Autodesk Fusion 360 part; units mm, degrees
sketch "Sketch1" plane through (0, 0, 0) normal (0, 1, 0) x (1, 0, 0)
  line L0 (17.145, 0) -> (68.58, 0)
  line L1 (91.44, 22.86) -> (91.44, 109.855)
  line L2 (74.295, 127) -> (22.86, 127)
  line L3 (0, 104.14) -> (0, 17.145)
  circle A0 centre (12.7, 31.75) radius 1.905
  circle A1 centre (78.74, 95.25) radius 1.905
  circle A2 centre (78.74, 31.75) radius 1.905
  circle A3 centre (12.7, 95.25) radius 1.905
  circle A4 centre (28.525, 20.96) radius 1.375
  circle A5 centre (62.915, 20.96) radius 1.375
  circle A6 centre (62.915, 106.04) radius 1.375
  circle A7 centre (28.525, 106.04) radius 1.375
  line L4 (22.86, 127) -> (0, 104.14)
  line L5 (91.44, 109.855) -> (74.295, 127)
  line L6 (68.58, 0) -> (91.44, 22.86)
  line L7 (17.145, 0) -> (0, 17.145)
  point P0 (91.44, 0)
  point P1 (91.44, 127)
  point P2 (0, 127)
  dimension "d1" = 91.44
  dimension "d8" = 2.75
  dimension "d63" = 22.86
  dimension "d64" = 22.86
  dimension "d65" = 17.145
  dimension "d66" = 17.145
  dimension "d67" = 22.86
  dimension "d68" = 22.86
  dimension "d69" = 17.145
  dimension "d70" = 17.145
extrude "Extrude5" add sketch "Sketch1" along normal blind 2.794
equation "d64 = d63"
equation "d66 = d65"
equation "d68 = d67"
equation "d70 = d69"
Check sheet for the modelled part. Datum: model origin and axes. Units: mm. Coordinates: 2 decimals unless noted, no trailing zeros. Loops run counter-clockwise (first coordinate to the right, second up) from the corner with the lowest first, then second, coordinate; pieces in that order, holes last. Notation, with made-up numbers: (-17, -35) -> (30, -35) arc R25 ccw to (30, -12) -> close; hole circle Ø11 at (14, 64). An arc over 180 degrees is marked (long way). Write item = value, one per line. Start each with the question number.
1. Depth check by flat-ended pin: P1, Ø2.5, axis at x = 28.525, z = -106.04, coming from the +Y side. Enter the tip coordinate at first touch or a pass-through.
2. Material ranges on line 1 (X direction, y = 1.65, z = -31.75) (3 decimals); line 2 (Z direction, x = 12.7, y = 1.9) (3 decimals); line 3 (X direction, y = 1, z = -20.96), recorded low to high.
3. Section check D-D on z = -117. Record the cut outline in (x, y) (3 decimals).
4. Draft check along X on faces 1 (the flat face through (79.85, 1.38, -11.27)), 2 (the cylindrical face through (77.3, 1.4, -94)), 3 (the flat face through (8.693, 1.377, -8.452)). Enter one of: released by +X, released by -X, zero draft, split by the parting line, or undercut.
5. Section check C-C on x = 12.7. Record the cut outline in (y, z) (3 decimals).
6. Section check A-A on z = -31.75. Record the cut outline in (x, y) (3 decimals).
7. Section check B-B on y = 1.9. Give the number of separate pieces and of enclosed holes in the cut face, then the cut area to 3 significant figures.
Responses:
q1.P1 = through
q2.line_1 = 0 to 10.795, 14.605 to 76.835, 80.645 to 91.44
q2.line_2 = -116.84 to -97.155, -93.345 to -33.655, -29.845 to -4.445
q2.line_3 = 0 to 27.15, 29.9 to 61.54, 64.29 to 89.54
q3.outline = (12.86, 0) -> (84.295, 0) -> (84.295, 2.794) -> (12.86, 2.794) -> close
q4.face_1 = released by +X
q4.face_2 = undercut
q4.face_3 = released by -X
q5.outline = (0, -116.84) -> (2.794, -116.84) -> (2.794, -97.155) -> (0, -97.155) -> close; (0, -93.345) -> (2.794, -93.345) -> (2.794, -33.655) -> (0, -33.655) -> close; (0, -29.845) -> (2.794, -29.845) -> (2.794, -4.445) -> (0, -4.445) -> close
q6.outline = (0, 0) -> (10.795, 0) -> (10.795, 2.794) -> (0, 2.794) -> close; (14.605, 0) -> (76.835, 0) -> (76.835, 2.794) -> (14.605, 2.794) -> close; (80.645, 0) -> (91.44, 0) -> (91.44, 2.794) -> (80.645, 2.794) -> close
q7.separate_pieces = 1
q7.enclosed_holes = 8
q7.area = 10,700 mm2
